Autodesk Inventor part; units mm, degrees
ref_plane "YZ Plane" through (0, 0, 0) normal (1, 0, 0) x (0, 1, 0)
ref_plane "XZ Plane" through (0, 0, 0) normal (0, 1, 0) x (-1, 0, 0)
ref_plane "XY Plane" through (0, 0, 0) normal (0, 0, 1) x (1, 0, 0)
sketch "Sketch1" plane through (0, 0, 0) normal (0, 0, 1) x (1, 0, 0)
  line L0 (-71.12, 0) -> (71.12, 0)
  line L1 (0, -71.12) -> (0, 71.12)
  circle A0 centre (0, 0) radius 50.8
  dimension "d0" = 101.6
extrude "Extrusion1" add sketch "Sketch1" against normal blind 19.05
sketch "Sketch2" plane through (0, 0, 0) normal (0, 0, 1) x (1, 0, 0)
  circle A0 centre (0, 0) radius 50.8
  circle A1 centre (0, 0) radius 30.1625
  dimension "d3" = 60.325
extrude "Extrusion2" add sketch "Sketch2" along normal blind 4.7625 contours A1
sketch "Sketch3" plane through (0, 0, 0) normal (0, 0, 1) x (1, 0, 0)
  circle A0 centre (0, 0) radius 30.1625
  point P0 (0, 44.45)
  point P1 (-44.45, 0)
  point P2 (0, -44.45)
  point P3 (44.45, 0)
  dimension "d8" = 360
  dimension "d35" = 88.9
hole "Hole1" at (0, 44.45, 0) at (-44.45, 0, 0) at (0, -44.45, 0) at (44.45, 0, 0) direction (0, 0, -1) diameter 6.4008 end through all
sketch "Sketch5" plane through (0, 0, -19.05) normal (0, 0, -1) x (-1, 0, 0)
  circle A0 centre (0, 0) radius 50.8
  circle A1 centre (0, 0) radius 38.1
  dimension "d17" = 76.2
extrude "Extrusion3" add sketch "Sketch5" along normal blind 50.8 draft -15 contours A1
sketch "Sketch6" plane through (0, 0, -69.85) normal (0, 0, -1) x (-1, 0, 0)
  circle A0 centre (0, 0) radius 24.4882
  point P0 (0, 17.4625)
  point P1 (-15.123, 8.7313)
  point P2 (-15.123, -8.7312)
  point P3 (0, -17.4625)
  point P4 (15.123, -8.7313)
  point P5 (15.123, 8.7312)
  dimension "d22" = 360
  dimension "d24" = 17.4625
hole "Hole2" at (0, 17.4625, -69.85) at (15.123, 8.7313, -69.85) at (15.123, -8.7312, -69.85) at (0, -17.4625, -69.85) at (-15.123, -8.7313, -69.85) at (-15.123, 8.7312, -69.85) direction (0, 0, 1) diameter 3.683 depth 12.7 tip angle 118
sketch "Sketch7" plane through (0, 0, 4.7625) normal (0, 0, 1) x (1, 0, 0)
  circle A0 centre (0, 0) radius 30.1625
  circle A1 centre (0, 0) radius 6.35
  dimension "d32" = 12.7
extrude "Extrusion4" cut sketch "Sketch7" against normal through all contours A1
properties part number "wheel_hub"
Input: part model. Units: mm. Frame: model coordinates. A direction names the side the tool comes from. Coordinates: 2 decimals unless noted, no trailing zeros. Loops run counter-clockwise (first coordinate to the right, second up) from the corner with the lowest first, then second, coordinate; pieces in that order, holes last. Notation, with made-up numbers: M 60,2 L 109,2 A17 ccw 109,12 Z; hole C 14.25,34.5 d3. An arc over 180 degrees is marked long. One line per item, written item: value.
(1) Section B-B (z = -9). Output: boundary loops of the cut face in (x, y).
Filled in:
outline: C 0,0 d101.6; hole C -44.45,0 d6.4; hole C 0,0 d12.7; hole C 0,-44.45 d6.4; hole C 0,44.45 d6.4; hole C 44.45,0 d6.4
(2) Pull-direction query (Y, two-part tool) for faces 1 (the flat face through (-7, 0, 4.762)), 2 (the cylindrical face through (13.3, -9, -63.4)), 3 (the cylindrical face through (-11.012, -49.592, -9.392)); classes: +Y half, -Y half, draft (parallel to the pull), parting line (faces both ways), or undercut.
Filled in:
face 1: draft
face 2: undercut
face 3: parting line
(3) Line query: line 1 along Y through (x, z) = (15.5, -61); line 2 along Z through (x, y) = (40, -4.5); line 3 along X through (y, z) = (-4.5, -17). Output: solid intervals per line, ascending. Write a range as from..to.
Filled in:
line 1: -21.94..-10.53, -6.93..6.93, 10.53..21.94
line 2: -19.05..0
line 3: -50.6..-4.48, 4.48..50.6
(4) Section A-A (y = 0). Output: boundary loops of the cut face in (x, z).
Filled in:
outline: M -50.8,-19.05 L -47.65,-19.05 L -47.65,0 L -50.8,0 Z; M -41.25,-19.05 L -38.1,-19.05 L -24.49,-69.85 L -6.35,-69.85 L -6.35,4.76 L -30.16,4.76 L -30.16,0 L -41.25,0 Z; M 6.35,-69.85 L 24.49,-69.85 L 38.1,-19.05 L 41.25,-19.05 L 41.25,0 L 30.16,0 L 30.16,4.76 L 6.35,4.76 Z; M 47.65,-19.05 L 50.8,-19.05 L 50.8,0 L 47.65,0 Z
(5) Section C-C (x = 44.45). Output: boundary loops of the cut face in (y, z).
Filled in:
outline: M -24.59,-19.05 L -3.2,-19.05 L -3.2,0 L -24.59,0 Z; M 3.2,-19.05 L 24.59,-19.05 L 24.59,0 L 3.2,0 Z
(6) Section D-D (z = -59). Output: boundary loops of the cut face in (x, y), and give its area (3 significant figures).
Filled in:
outline: C 0,0 d54.79; hole C -15.12,-8.73 d3.68; hole C -15.12,8.73 d3.68; hole C 0,0 d12.7; hole C 0,-17.46 d3.68; hole C 0,17.46 d3.68; hole C 15.12,-8.73 d3.68; hole C 15.12,8.73 d3.68
area: 2,170 mm^2
(7) Pin query (flat end, axial travel): pin 1 (10 mm diameter, centred on x = 0, y = -44.45, fed in from +Z); pin 2 (1.5 mm diameter, centred on y = -23.5, z = -29, fed in from +X); pin 3 (5 mm diameter, centred on x = -2.5, z = -31.5, fed in from +Y). Return the tip coordinate at first contact, or that it passes through.
Filled in:
pin 1: z = 0
pin 2: x = 27.22
pin 3: y = 35.36
(8) Reachability of faces 4 (the flat face through (22, -22, 0)), 5 (the cylindrical face through (-0.55, 19.22, -63.41)), 6 (the cylindrical face through (-47.623, 0.417, -9.658)) from +Z, -Z, +X, -X, +Y, -Y: full face, straight path, thin tool, end or side. Return the list, or none.
Filled in:
face 4: +Z
face 5: -Z
face 6: +Z, -Z
